The figure shows three views and two pictorial views of one solid part (mm, origin at its lowest corner). Answer the questions. A direction names the side the tool comes from. Round coordinates to 2 decimals unless told otherwise and drop trailing zeros. Loops run counter-clockwise (first coordinate to the right, second up) from the corner with the lowest first, then second, coordinate; pieces in that order, holes last. Notation, with made-up numbers: (31, 20) -> (82, 20) arc R6 cw to (82, 24) -> close; hole circle Ø6 at (86, 24.5). An arc over 180 degrees is marked (long way). Write item = value, one per line. Start each with the question number.
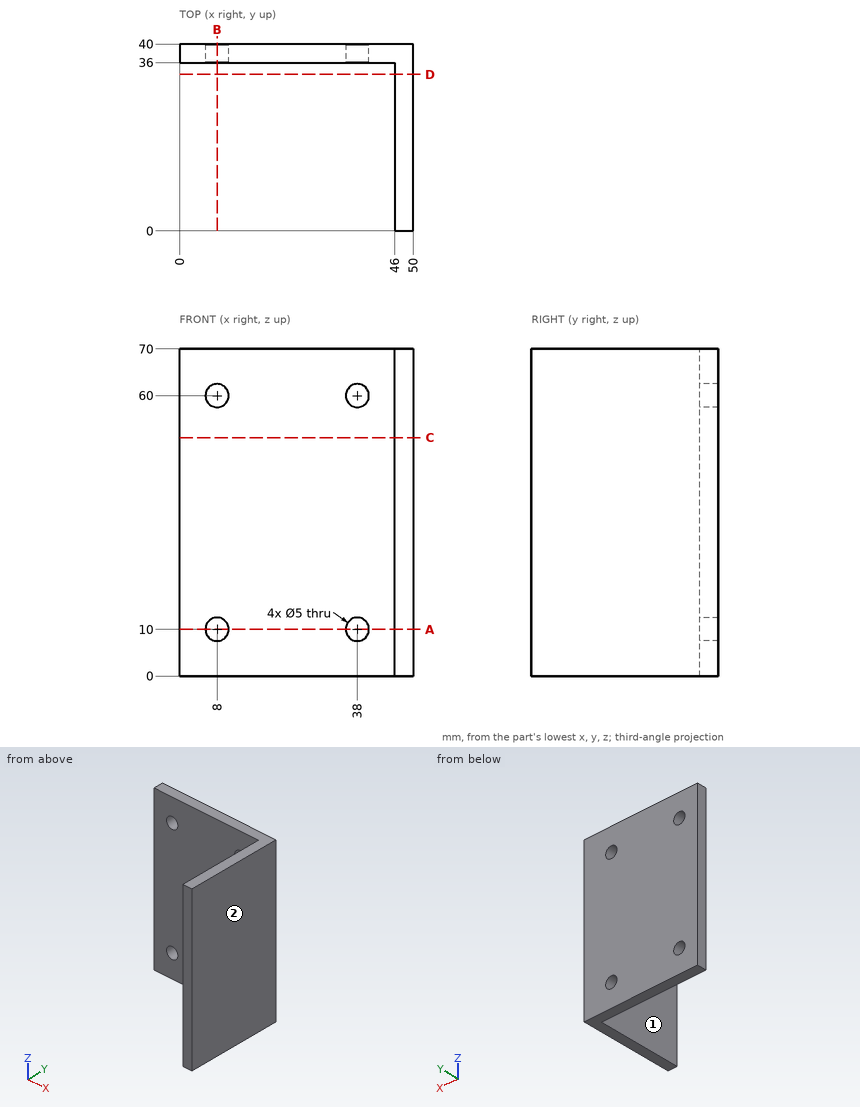
Item 1: Section C-C (z = 51) is taken. Determine the outline of the cut face in (x, y), then the cut area to 3 significant figures.
Item 2: Find the intervals of material crossed by line 1 along Z through (x, y) = (8, 37); line 2 along Y through (x, z) = (40.5, 13); line 3 along X through (y, z) = (34, 63), in increasing order. Write a range as [from, to].
Item 3: Section D-D (y = 33.5) is taken. Determine the outline of the cut face in (x, z).
Item 4: A tool of negligible diameter and unlimited length cuts with its end or side. For the marked faces 1 and 2, from which of +Z, -Z, +X, -X, +Y, -Y can it reach the whole face along a straight path? Write none if from no direction.
Item 5: Flat-ended cylindrical pins translate along their axes: pin 1 (12 mm diameter, centred on y = 23.5, z = 30, fed in from -X); pin 2 (1 mm diameter, centred on x = 37, z = 55.5, fed in from -Y). Find the tip coordinate at first contact, or state that the pin passes through.
Item 6: Section A-A (z = 10) is taken. Determine the outline of the cut face in (x, y).
Item 7: Section B-B (x = 8) is taken. Determine the outline of the cut face in (y, z), then the cut area to 3 significant figures.
Worked answers:
q1.outline = (0, 36) -> (46, 36) -> (46, 0) -> (50, 0) -> (50, 40) -> (0, 40) -> close
q1.area = 344 mm2
q2.line_1 = [0, 7.5], [12.5, 57.5], [62.5, 70]
q2.line_2 = [36, 40]
q2.line_3 = [46, 50]
q3.outline = (46, 0) -> (50, 0) -> (50, 70) -> (46, 70) -> close
q4.face_1 = +Z, -Z, -X, -Y
q4.face_2 = +Z, -Z, +X, +Y, -Y
q5.pin_1 = 46
q5.pin_2 = 36
q6.outline = (0, 36) -> (5.5, 36) -> (5.5, 40) -> (0, 40) -> close; (10.5, 36) -> (35.5, 36) -> (35.5, 40) -> (10.5, 40) -> close; (40.5, 36) -> (46, 36) -> (46, 0) -> (50, 0) -> (50, 40) -> (40.5, 40) -> close
q7.outline = (36, 0) -> (40, 0) -> (40, 7.5) -> (36, 7.5) -> close; (36, 12.5) -> (40, 12.5) -> (40, 57.5) -> (36, 57.5) -> close; (36, 62.5) -> (40, 62.5) -> (40, 70) -> (36, 70) -> close
q7.area = 240 mm2
